Source: three-view drawing plus pictorial views. Frame: mm from the lowest corner of the part. Give positions to 0.01 mm unless a question says otherwise; leave off trailing zeros. Order: outer loops, then holes, each group sorted by start corner. A loop starts at its lowest first (then second) coordinate and runs counter-clockwise, first axis right, second up. Notation, with made-up numbers: (11.5, 32) - (48.5, 32) arc R31 cw to (48.5, 62) - close; hole circle Ø2 at (-13.75, -38). An arc over 180 degrees is marked (long way). Answer in a Markdown table with one row per item. Add a question column.
1. Section query D-D on z = 39. Return loops of the section in (x, y).
2. Contact query for a flat-ended pin moving along its axis: pin 1 (4 mm diameter, centred on x = 69.342, z = 40.005, fed in from +Y). Output: stop coordinate, or through.
3. Section query C-C on x = 12.7. Count the separate pieces of the cut face and the enclosed holes in it, and give its area (3 significant figures).
4. Section query B-B on z = 52.07. Return loops of the section in (x, y).
5. Ray query, line 1 (Z direction, x = 12.7, y = 3.25) (1 decimal); line 2 (Z direction, x = 50.8, y = 1.5) (1 decimal); line 3 (X direction, y = 1, z = 41) (1 decimal). Return the intervals inside material, ascending. Write a range as [from, to].
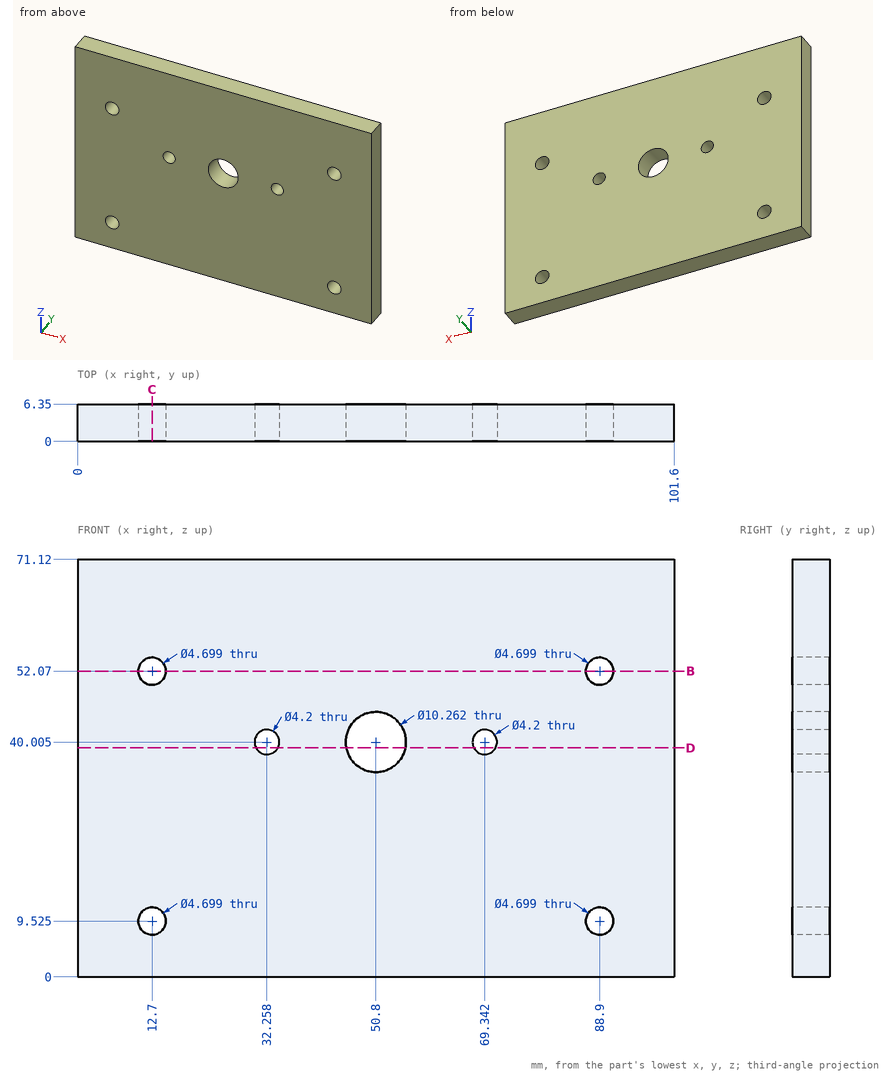
Answer:
| question | item | result |
|---|---|---|
| 1 | outline | (0, 0) - (30.41, 0) - (30.41, 6.35) - (0, 6.35) - close; (34.1, 0) - (45.77, 0) - (45.77, 6.35) - (34.1, 6.35) - close; (55.83, 0) - (67.5, 0) - (67.5, 6.35) - (55.83, 6.35) - close; (71.19, 0) - (101.6, 0) - (101.6, 6.35) - (71.19, 6.35) - close |
| 2 | pin 1 | passes through |
| 3 | separate pieces | 3 |
| 3 | enclosed holes | 0 |
| 3 | area | 392 mm² |
| 4 | outline | (0, 0) - (10.35, 0) - (10.35, 6.35) - (0, 6.35) - close; (15.05, 0) - (86.55, 0) - (86.55, 6.35) - (15.05, 6.35) - close; (91.25, 0) - (101.6, 0) - (101.6, 6.35) - (91.25, 6.35) - close |
| 5 | line 1 | z = [0, 7.2], [11.9, 49.7], [54.4, 71.1] |
| 5 | line 2 | z = [0, 34.9], [45.1, 71.1] |
| 5 | line 3 | x = [0, 30.4], [34.1, 45.8], [55.8, 67.5], [71.2, 101.6] |
